Verification items for the finished model (mm, model axes). Coordinates: 2 decimals unless noted, no trailing zeros. Answer as a JSON object with one key per item and string values. Group by question number.
Q1. Cross-section at A-A on y = 2.6. Give the number of separate pieces and of enclosed holes in the cut face, and give its area (3 significant figures).
Q2. Gauge pin test, flat ends, axial feed: pin 1 Ø5 at (x, z) = (-65, -1) entering from +Y (3 decimals); pin 2 Ø7 at (x, z) = (-475, -1) entering from +Y (3 decimals). Record the tip position at first contact, or that the pin passes through.
Q3. Scan lines: L1, parallel to Z at x = 55, y = 1.55; L2, parallel to Z at x = -475, y = 0.2. Record each from-to range of solid material in increasing order.
```python
from build123d import *

# Parameters (mm, degrees)
SKETCH1_W                    = 960
SKETCH1_H                    = 12
BOSS_EXTRUDE1_DEPTH          = 3.175
CSK_FOR_M4_SFHCS1_AT_2_COUNT = 2
CSK_FOR_M4_SFHCS1_AT_2_PITCH = 570
CSK_FOR_M4_SFHCS1_AT_3_COUNT = 2
CSK_FOR_M4_SFHCS1_AT_3_PITCH = 540
CSK_FOR_M4_SFHCS1_AT_4_COUNT = 2
CSK_FOR_M4_SFHCS1_AT_4_PITCH = 430
CSK_FOR_M4_SFHCS1_AT_5_COUNT = 2
CSK_FOR_M4_SFHCS1_AT_5_PITCH = 400
CSK_FOR_M4_SFHCS1_AT_6_COUNT = 2
CSK_FOR_M4_SFHCS1_AT_6_PITCH = 950
M4X0_7_TAPPED_HOLE2_D        = 3.3


with BuildPart() as part:
    # Sketch1 → Boss-Extrude1 (new body)
    with BuildSketch(Plane(origin=(0, 0, 0), x_dir=(1, 0, 0), z_dir=(0, 1, 0))):
        Rectangle(SKETCH1_W, SKETCH1_H)
    extrude(amount=BOSS_EXTRUDE1_DEPTH)

    # Sketch3 → CSK for M4 SFHCS1 (revolve, cut)
    with BuildSketch(Plane(origin=(475, 3.175, -1), x_dir=(0, 0, 1), z_dir=(1, 0, 0))):
        Polygon((0, 0), (0, 3.175), (2.25, 3.175), (2.25, 2.23), (4.48, 0), align=None)
    csk_for_m4_sfhcs1 = revolve(axis=Axis((475, 9.525, -1), (0, -1, 0)), mode=Mode.SUBTRACT)

    # CSK for M4 SFHCS1 at 2: CSK for M4 SFHCS1 ×2
    with Locations(*[(-i * CSK_FOR_M4_SFHCS1_AT_2_PITCH, 0, 0) for i in range(1, CSK_FOR_M4_SFHCS1_AT_2_COUNT)]):
        add(csk_for_m4_sfhcs1, mode=Mode.SUBTRACT)

    # CSK for M4 SFHCS1 at 3: CSK for M4 SFHCS1 ×2
    with Locations(*[(-i * CSK_FOR_M4_SFHCS1_AT_3_PITCH, 0, 0) for i in range(1, CSK_FOR_M4_SFHCS1_AT_3_COUNT)]):
        add(csk_for_m4_sfhcs1, mode=Mode.SUBTRACT)

    # CSK for M4 SFHCS1 at 4: CSK for M4 SFHCS1 ×2
    with Locations(*[(-i * CSK_FOR_M4_SFHCS1_AT_4_PITCH, 0, 0) for i in range(1, CSK_FOR_M4_SFHCS1_AT_4_COUNT)]):
        add(csk_for_m4_sfhcs1, mode=Mode.SUBTRACT)

    # CSK for M4 SFHCS1 at 5: CSK for M4 SFHCS1 ×2
    with Locations(*[(-i * CSK_FOR_M4_SFHCS1_AT_5_PITCH, 0, 0) for i in range(1, CSK_FOR_M4_SFHCS1_AT_5_COUNT)]):
        add(csk_for_m4_sfhcs1, mode=Mode.SUBTRACT)

    # CSK for M4 SFHCS1 at 6: CSK for M4 SFHCS1 ×2
    with Locations(*[(-i * CSK_FOR_M4_SFHCS1_AT_6_PITCH, 0, 0) for i in range(1, CSK_FOR_M4_SFHCS1_AT_6_COUNT)]):
        add(csk_for_m4_sfhcs1, mode=Mode.SUBTRACT)

    # M4x0.7 Tapped Hole2 (through all)
    with Locations(Plane(origin=(0, 3.175, 0), x_dir=(1, 0, 0), z_dir=(0, 1, 0))):
        with Locations((-85, 1), (-75, 1), (55, 1), (65, 1), (175, 1), (375, 1), (-385, 1), (-185, 1)):
            Hole(M4X0_7_TAPPED_HOLE2_D / 2)


solid = part.part
```
Computed values:
{
 "1": {"separate pieces": "1", "enclosed holes": "14", "area": "11,200 mm²"},
 "2": {"pin 1": "stops at y = 1.195", "pin 2": "stops at y = 2.195"},
 "3": {"L1": "z = -6 to -2.65, 0.65 to 6", "L2": "z = -6 to -3.25, 1.25 to 6"}
}
